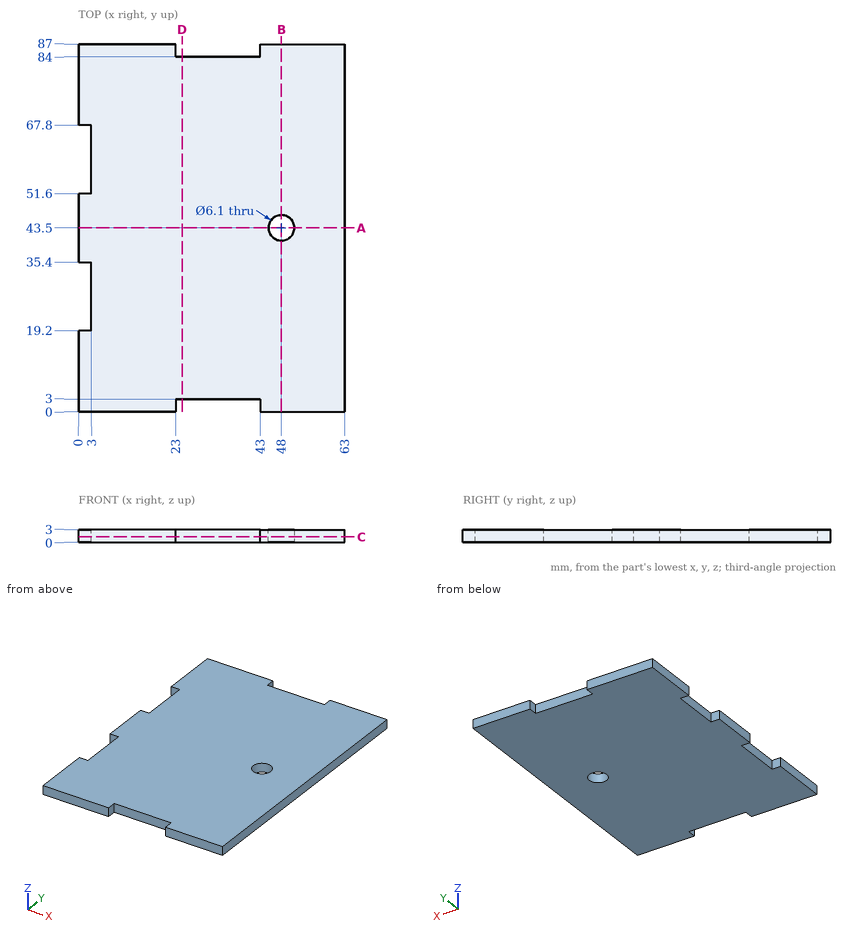
Verification items for this drawing (mm, ordinates from the low corner). Give positions to 0.01 mm unless a question says otherwise; leave off trailing zeros. Write each loop counter-clockwise with the first axis right and the second up, starting at its lowest first coordinate (ties: lowest second). Pieces come first, ordered by that corner, then holes. Notation, with made-up numbers: (68.5, 59) - (105.5, 59) arc R22 cw to (105.5, 73) - close; hole circle Ø9 at (7.5, 68). An arc over 180 degrees is marked (long way). Answer as CSV lines item,"result". Start each with the question number.
1. Sectioned sample at A-A (y = 43.5). Record the boundary of the cut face in (x, z), then the cut area to 3 significant figures.
2. Depth check by flat-ended pin: pin 1 (1.5 mm diameter, centred on y = 1, z = 2, fed in from -X); pin 2 (5.5 mm diameter, centred on x = 48, y = 43.5, fed in from +Z). Enter the tip coordinate at first touch or a pass-through.
3. Sectioned sample at C-C (z = 1.3). Record the boundary of the cut face in (x, y), then the cut area to 3 significant figures.
4. Sectioned sample at B-B (x = 48). Record the boundary of the cut face in (y, z), then the cut area to 3 significant figures.
5. Sectioned sample at D-D (x = 24.5). Record the boundary of the cut face in (y, z), then the cut area to 3 significant figures.
6. Thickness scan on line 1 (X direction, y = 43.5, z = 0.9); line 2 (Y direction, x = 48, z = 2); line 3 (X direction, y = 62.5, z = 2.9). Record the ranges inside material, lowest first.
Derived:
1,outline,"(0, 0) - (44.95, 0) - (44.95, 3) - (0, 3) - close; (51.05, 0) - (63, 0) - (63, 3) - (51.05, 3) - close"
1,area,"171 mm²"
2,pin 1,"x = 0"
2,pin 2,"through"
3,outline,"(0, 0) - (23, 0) - (23, 3) - (43, 3) - (43, 0) - (63, 0) - (63, 87) - (43, 87) - (43, 84) - (23, 84) - (23, 87) - (0, 87) - (0, 67.8) - (3, 67.8) - (3, 51.6) - (0, 51.6) - (0, 35.4) - (3, 35.4) - (3, 19.2) - (0, 19.2) - close; hole circle Ø6.1 at (48, 43.5)"
3,area,"5,230 mm²"
4,outline,"(0, 0) - (40.45, 0) - (40.45, 3) - (0, 3) - close; (46.55, 0) - (87, 0) - (87, 3) - (46.55, 3) - close"
4,area,"243 mm²"
5,outline,"(3, 0) - (84, 0) - (84, 3) - (3, 3) - close"
5,area,"243 mm²"
6,line 1,"0 to 44.95, 51.05 to 63"
6,line 2,"0 to 40.45, 46.55 to 87"
6,line 3,"3 to 63"
